```python
from build123d import *

# Parameters (mm, degrees)
F0_W     = 546.735
F0_H     = 347.5
F1_DEPTH = 3
F2_W     = 408.735
F2_H     = 3
F3_DEPTH = 37.5


with BuildPart() as f1:
    # F0 (on Front) → F1 (new body)
    with BuildSketch(Plane.XZ):
        Rectangle(F0_W, F0_H)
    extrude(amount=F1_DEPTH)

    # F2 (on face) → F3 (join)
    with BuildSketch(Plane(origin=(0, 0, -173.75), x_dir=(1, 0, 0), z_dir=(0, 0, -1))):
        with Locations((0, 1.5)):
            Rectangle(F2_W, F2_H)
    extrude(amount=F3_DEPTH)


solid = f1.part
```
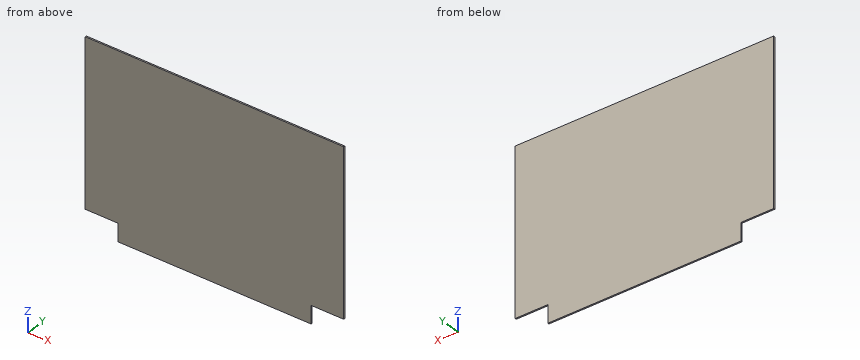
Check sheet for the modelled part. Datum: model origin and axes. Units: mm. Round coordinates to 2 decimals unless told otherwise and drop trailing zeros. Write each loop counter-clockwise with the first axis right and the second up, starting at its lowest first coordinate (ties: lowest second). Pieces come first, ordered by that corner, then holes. Notation, with made-up numbers: M 73.5,-39.5 L 120.5,-39.5 A29 ccw 120.5,-10.5 Z; hole C 44,-35 d5. An arc over 180 degrees is marked long. Write item = value, one per line. Start each with the question number.
1. Gauge pin test, flat ends, axial feed: pin 1 (1.5 mm diameter, centred on y = -2, z = -190, fed in from -X); pin 2 (1.5 mm diameter, centred on x = 251, y = -1.5, fed in from -Z). Record the tip position at first contact, or that the pin passes through.
2. Section check B-B, the plane x = 216.5. Record the cut outline in (y, z), then the cut area to 3 significant figures.
3. Section check A-A, the plane y = -2.5. Record the cut outline in (x, z), then the cut area to 3 significant figures.
4. Section check C-C, the plane z = -186. Record the cut outline in (x, y).
5. Scan lines: line 1 (Z direction, x = -238, y = -2.8); line 2 (X direction, y = -0.3, z = -182). Record each from-to range of solid material in increasing order. Write a range as [from, to].
Results found:
q1.pin_1 = -204.37
q1.pin_2 = -173.75
q2.outline = M -3,-173.75 L 0,-173.75 L 0,173.75 L -3,173.75 Z
q2.area = 1,040 mm^2
q3.outline = M -273.37,-173.75 L -204.37,-173.75 L -204.37,-211.25 L 204.37,-211.25 L 204.37,-173.75 L 273.37,-173.75 L 273.37,173.75 L -273.37,173.75 Z
q3.area = 205,000 mm^2
q4.outline = M -204.37,-3 L 204.37,-3 L 204.37,0 L -204.37,0 Z
q5.line_1 = [-173.75, 173.75]
q5.line_2 = [-204.37, 204.37]
